Check sheet for the modelled part. Datum: model origin and axes. Units: mm. A direction names the side the tool comes from. Give positions to 0.01 mm unless a question says otherwise; leave off trailing zeros. Write each loop counter-clockwise with the first axis right and the second up, starting at its lowest first coordinate (ties: lowest second). Pieces come first, ordered by that corner, then holes.
Autodesk Fusion 360 part; units mm, degrees
sketch "Sketch3" plane through (0, 0, 0) normal (0, 0, 1) x (1, 0, 0)
  line L0 (0, 0) -> (32, 0)
  line L1 (32, 0) -> (32, 32)
  line L2 (32, 32) -> (0, 32)
  line L3 (0, 32) -> (0, 0)
  line L4 (-0.5, 32.5) -> (-0.5, -0.5)
  line L5 (-0.5, -0.5) -> (32.5, -0.5)
  line L6 (32.5, -0.5) -> (32.5, 32.5)
  line L7 (32.5, 32.5) -> (-0.5, 32.5)
  line L8 (70, 32) -> (38, 32)
  line L9 (38, 32) -> (38, 0)
  line L10 (37.5, -0.5) -> (70.5, -0.5)
  line L11 (70.5, 32.5) -> (37.5, 32.5)
  line L12 (70, 0) -> (70, 32)
  line L13 (70.5, -0.5) -> (70.5, 32.5)
  line L14 (38, 0) -> (70, 0)
  line L15 (37.5, 32.5) -> (37.5, -0.5)
  line L16 (108, 32) -> (76, 32)
  line L17 (76, 32) -> (76, 0)
  line L18 (75.5, -0.5) -> (108.5, -0.5)
  line L19 (108.5, 32.5) -> (75.5, 32.5)
  line L20 (108, 0) -> (108, 32)
  line L21 (108.5, -0.5) -> (108.5, 32.5)
  line L22 (76, 0) -> (108, 0)
  line L23 (75.5, 32.5) -> (75.5, -0.5)
  line L24 (38, 32) -> (70, 0)
  line L25 (70, 32) -> (38, 0)
  line L26 (118, -10) -> (-10, -10)
  line L27 (-10, -10) -> (-10, 42)
  line L28 (-10, 42) -> (118, 42)
  line L29 (118, 42) -> (118, -10)
  line L30 (118, -10) -> (-10, 42) construction
  line L31 (-10, -10) -> (118, 42) construction
  circle A0 centre (3, 26) radius 2.05
  circle A1 centre (3, 26) radius 3.55
  circle A2 centre (29, 26) radius 3.55
  circle A3 centre (29, 26) radius 2.05
  circle A4 centre (29, 6) radius 2.05
  circle A5 centre (29, 6) radius 3.55
  circle A6 centre (3, 6) radius 2.05
  circle A7 centre (3, 6) radius 3.55
  circle A8 centre (67, 6) radius 2.05
  circle A9 centre (67, 6) radius 3.55
  circle A10 centre (41, 6) radius 2.05
  circle A11 centre (41, 6) radius 3.55
  circle A12 centre (67, 26) radius 2.05
  circle A13 centre (67, 26) radius 3.55
  circle A14 centre (41, 26) radius 2.05
  circle A15 centre (41, 26) radius 3.55
  circle A16 centre (105, 6) radius 2.05
  circle A17 centre (105, 6) radius 3.55
  circle A18 centre (79, 6) radius 2.05
  circle A19 centre (79, 6) radius 3.55
  circle A20 centre (105, 26) radius 2.05
  circle A21 centre (105, 26) radius 3.55
  circle A22 centre (79, 26) radius 2.05
  circle A23 centre (79, 26) radius 3.55
  line L32 (3, 22.45) -> (-0.5, 22.45)
  line L33 (-0.5, 22.45) -> (-0.5, 9.55)
  line L34 (-0.5, 9.55) -> (3, 9.55)
  line L35 (3, 9.55) -> (3, 22.45)
  line L36 (41, 22.45) -> (37.5, 22.45)
  line L37 (41, 9.55) -> (41, 22.45)
  line L38 (37.5, 9.55) -> (41, 9.55)
  line L39 (37.5, 22.45) -> (37.5, 9.55)
  line L40 (79, 22.45) -> (75.5, 22.45)
  line L41 (79, 9.55) -> (79, 22.45)
  line L42 (75.5, 9.55) -> (79, 9.55)
  line L43 (75.5, 22.45) -> (75.5, 9.55)
  circle A24 centre (-6, 38) radius 1.55
  circle A25 centre (-6, 38) radius 3.05
  circle A26 centre (54, 38) radius 1.55
  circle A27 centre (54, 38) radius 3.05
  circle A28 centre (114, 38) radius 1.55
  circle A29 centre (114, 38) radius 3.05
  circle A30 centre (-6, -6) radius 1.55
  circle A31 centre (-6, -6) radius 3.05
  circle A32 centre (54, -6) radius 1.55
  circle A33 centre (54, -6) radius 3.05
  circle A34 centre (114, -6) radius 1.55
  circle A35 centre (114, -6) radius 3.05
  line L44 (121, -20) -> (-13, -20)
  line L45 (-13, -20) -> (-13, 52)
  line L46 (-13, 52) -> (121, 52)
  line L47 (121, 52) -> (121, -20)
  line L48 (121, -20) -> (-13, 52) construction
  line L49 (-13, -20) -> (121, 52) construction
  circle A36 centre (-6, 48) radius 1.55
  circle A37 centre (114, 48) radius 1.55
  circle A38 centre (114, -16) radius 1.55
  circle A39 centre (-6, -16) radius 1.55
  line L50 (118, 15) -> (-10, 15)
  line L51 (-10, 15) -> (-10, 17)
  line L52 (-10, 17) -> (118, 17)
  line L53 (118, 17) -> (118, 15)
  line L54 (118, 15) -> (-10, 17) construction
  line L55 (-10, 15) -> (118, 17) construction
  line L56 (-10, -10) -> (118, -10)
  line L57 (118, -10) -> (118, -12)
  line L58 (118, -12) -> (-10, -12)
  line L59 (-10, -12) -> (-10, -10)
  line L60 (-10, 42) -> (118, 42)
  line L61 (118, 42) -> (118, 44)
  line L62 (118, 44) -> (-10, 44)
  line L63 (-10, 44) -> (-10, 42)
  point P0 (38, 0)
  point P1 (76, 0)
  point P2 (54, 16)
  point P3 (54, 16)
  point P4 (54, 16)
  dimension "d57" = 32
  dimension "d58" = 32
  dimension "d59" = 0.5
  dimension "d62" = 76
  dimension "d63" = 0
  dimension "d66" = 10
  dimension "d67" = 10
  dimension "d68" = 4.1
  dimension "d69" = 3
  dimension "d70" = 6
  dimension "d71" = 7.1
  dimension "d74" = 26
  dimension "d75" = 0
  dimension "d78" = 0
  dimension "d79" = -20
  dimension "d82" = 76
  dimension "d83" = 0
  dimension "d84" = 3.5
  dimension "d85" = 12.9
  dimension "d86" = 9.55
  dimension "d89" = 76
  dimension "d90" = 0
  dimension "d95" = 4
  dimension "d96" = 4
  dimension "d97" = 3.1
  dimension "d98" = 6.1
  dimension "d101" = 120
  dimension "d102" = 0
  dimension "d105" = 0
  dimension "d106" = -44
  dimension "d114" = 134
  dimension "d115" = 72
  dimension "d116" = 3.1
  dimension "d117" = 7
  dimension "d118" = 4
  dimension "d121" = 120
  dimension "d122" = 0
  dimension "d125" = 0
  dimension "d126" = -64
  dimension "d127" = 128
  dimension "d128" = 2
  dimension "d134" = 2
  dimension "d135" = 2
extrude "Extrude4" add sketch "Sketch3" along normal blind 1.5 contours L4 A7 | L4 L5 L6 L10 L13 L15 L18 L21 L23 L26 L27 L29 A5 A7 A9 A11 A17 A19 L33 L39 L43 L50 L56 | L6 A5 | L6 L15 L39 L50 L52 | L4 L27 L33 L50 L51 L52 | L4 L6 L7 L11 L13 L15 L19 L21 L23 L27 L28 L29 A1 A2 A13 A15 A21 A23 L33 L39 L43 L52 L60 | L6 A2 | L26 L56 L57 L58 L59 | L15 A11 | L4 A1 | L28 L60 L61 L62 L63 | L15 A15 | L21 L29 L50 L52 L53 | L21 A17 | L13 A9 | L13 L23 L43 L50 L52 | L21 A21 | L13 A13 | L23 A19 | L23 A23 | A25 | A26 | A27 | A29 | A31 | A32 | A33 | A35 | L44 L45 L46 L47
extrude "Extrude6" add sketch "Sketch3" along normal blind 4 contours L26 L56 L57 L58 L59 | L28 L60 L61 L62 L63
chamfer "Chamfer2" distance 2.5 angle 45 4 edges at (118, 43, 4) (118, -11, 4) (-10, -11, 4) (-10, 43, 4)
extrude "Extrude5" add sketch "Sketch3" along normal blind 2.5 contours L6 L15 L39 L50 L52 | L4 L27 L33 L50 L51 L52 | L21 L29 L50 L52 L53 | L13 L23 L43 L50 L52
chamfer "Chamfer1" distance 1 angle 45 8 edges at (118, 16, 2.5) (108.5, 16, 2.5) (75.5, 16, 2.5) (70.5, 16, 2.5) (37.5, 16, 2.5) (32.5, 16, 2.5) (-0.5, 16, 2.5) (-10, 16, 2.5)
equation "d71 = d68 + 3 mm"
equation "d98 = d97 + 3 mm"
equation "d115 = 52 mm + 20 mm"
equation "d116 = d97"
1) Scan lines: L1, parallel to Y at x = -6, z = 0.75; L2, parallel to X at y = 23, z = 1.05; L3, parallel to Y at x = 7.5, z = 3.3. Record each from-to range of solid material in increasing order.
2) Access from +Z, -Z, +X, -X, +Y, -Y to the whole of each face (thin tool, end or side, straight path). Record for faces 4 (the flat face through (-8.7, -11, 2.8)), 5 (the cylindrical face through (-7.14, -7.05, 0.74)), 6 (the flat face through (55, -12, 3)), 7 (the flat face through (55, 44, 3)), 8 (the flat face through (53, 42, 3)).
3) Sectioned sample at B-B on x = 100.5. Record the boundary of the cut face in (y, z).
4) Sectioned sample at D-D on x = -6. Give the number of separate pieces and of enclosed holes in the cut face, then the cut area to 3 significant figures.
5) Sectioned sample at A-A on y = -16. Record the boundary of the cut face in (x, z).
6) Gauge pin test, flat ends, axial feed: pin 1 (4 mm diameter, centred on x = 114, y = -6, fed in from -Z); pin 2 (1.6 mm diameter, centred on x = -6, y = 16, fed in from +Z); pin 3 (6 mm diameter, centred on x = 48.5, y = 35.5, fed in from +Z); pin 4 (1.5 mm diameter, centred on x = 26.5, z = 3, fed in from -Y). Record the tip position at first contact, or that the pin passes through.
7) Sectioned sample at C-C on y = 10.5. Record the boundary of the cut face in (x, z).
8) Draft check along X on faces 1 (the flat face through (-8.7, 43, 2.8)), 2 (the flat face through (53, 33, 1.5)), 3 (the cylindrical face through (112.45, 37.93, 0.74)). Enter one of: +X half, -X half, draft (parallel to the pull), parting line (faces both ways), or undercut.
Answers below:
1. L1: y = -20 to -17.55, -14.45 to -7.55, -4.45 to 36.45, 39.55 to 46.45, 49.55 to 52
1. L2: x = -13 to -0.5, 32.5 to 37.5, 70.5 to 75.5, 108.5 to 121
1. L3: y = -12 to -10, 42 to 44
2. face 4: +Z, -X, +Y, -Y
2. face 5: +Z, -Z
2. face 6: +Z, +X, -X, -Y
2. face 7: +Z, +X, -X, +Y
2. face 8: +Z, +X, -X
3. outline: (-20, 0) - (-0.5, 0) - (-0.5, 1.5) - (-10, 1.5) - (-10, 4) - (-12, 4) - (-12, 1.5) - (-20, 1.5) - close; (32.5, 0) - (52, 0) - (52, 1.5) - (44, 1.5) - (44, 4) - (42, 4) - (42, 1.5) - (32.5, 1.5) - close
4. separate pieces: 5
4. enclosed holes: 0
4. area: 101 mm2
5. outline: (-13, 0) - (-7.55, 0) - (-7.55, 1.5) - (-13, 1.5) - close; (-4.45, 0) - (112.45, 0) - (112.45, 1.5) - (-4.45, 1.5) - close; (115.55, 0) - (121, 0) - (121, 1.5) - (115.55, 1.5) - close
6. pin 1: stops at z = 0
6. pin 2: stops at z = 2.5
6. pin 3: stops at z = 1.5
6. pin 4: stops at y = -12
7. outline: (-13, 0) - (-0.5, 0) - (-0.5, 1.5) - (-13, 1.5) - close; (32.5, 0) - (37.5, 0) - (37.5, 1.5) - (32.5, 1.5) - close; (70.5, 0) - (75.5, 0) - (75.5, 1.5) - (70.5, 1.5) - close; (108.5, 0) - (121, 0) - (121, 1.5) - (108.5, 1.5) - close
8. face 1: -X half
8. face 2: draft
8. face 3: undercut
